Design review of the part built by this model. Coordinates are the model's own, in mm. Coordinates: 2 decimals unless noted, no trailing zeros. Order: outer loops, then holes, each group sorted by start corner. A loop starts at its lowest first (then second) coordinate and runs counter-clockwise, first axis right, second up. Notation, with made-up numbers: (87.5, 82.25) -> (110.5, 82.25) arc R9 ccw to (110.5, 94.25) -> close; hole circle Ø2 at (11.25, 73). An arc over 180 degrees is marked (long way). Use a Markdown table: item, result. Add a question column.
Q1. Insertion check: pin 1 (1 mm diameter, centred on y = 2, z = 43.5, fed in from +X); pin 2 (4 mm diameter, centred on x = -37.25, z = -37.25, fed in from +Y). Each pin has a flat end and moves straight along its axis. Give the tip position at first contact, or say it passes through.
Q2. Wall thickness on probe 1 along Z at (x, y) = (37.25, 1.3); probe 2 along Z at (x, y) = (-28, 0.9): over which ranges is each line inside the solid? List them lowest first.
Q3. Add section A-A (z = 37.25). State the section outline as (x, y) points (1 decimal), then the cut area to 3 significant figures.
Q4. Add section C-C (z = 0). State the section outline as (x, y) points (3 decimals), then the cut area to 3 significant figures.
Q5. Add section B-B (x = 0). State the section outline as (y, z) points (3 decimals), then the cut area to 3 significant figures.
Q6. Add section D-D (x = -37.25). State the section outline as (y, z) points (1 decimal).
from build123d import *

# Parameters (mm, degrees)
SKETCH1_W                                     = 98
SKETCH1_H                                     = 98
BOSS_EXTRUDE1_DEPTH                           = 3.175
SKETCH2_W                                     = 7.5
SKETCH2_H                                     = 7.5
CUT_EXTRUDE1_DEPTH                            = 70.369161917
F_4_CLEARANCE_HOLE1_D                         = 2.9464
M2_CLEARANCE_HOLE1_D                          = 2.2
CSK_FOR_4_FLAT_HEAD_MACHINE_SCREW1_AT_2_COUNT = 2
CSK_FOR_4_FLAT_HEAD_MACHINE_SCREW1_AT_2_PITCH = 74.5
CSK_FOR_4_FLAT_HEAD_MACHINE_SCREW1_AT_3_COUNT = 2
CSK_FOR_4_FLAT_HEAD_MACHINE_SCREW1_AT_3_PITCH = 105.358910397
CSK_FOR_4_FLAT_HEAD_MACHINE_SCREW1_AT_4_COUNT = 2
CSK_FOR_4_FLAT_HEAD_MACHINE_SCREW1_AT_4_PITCH = 74.5


with BuildPart() as part:
    # Sketch1 → Boss-Extrude1 (new body)
    with BuildSketch(Plane(origin=(0, 0, 0), x_dir=(1, 0, 0), z_dir=(0, 1, 0))):
        Rectangle(SKETCH1_W, SKETCH1_H)
    extrude(amount=BOSS_EXTRUDE1_DEPTH)

    # Sketch2 → Cut-Extrude1 (cut, through all)
    with BuildSketch(Plane(origin=(0, 3.175, 0), x_dir=(1, 0, 0), z_dir=(0, 1, 0))):
        with Locations((45.25, 45.25)):
            Rectangle(SKETCH2_W, SKETCH2_H)
        with Locations((-45.25, 45.25)):
            Rectangle(SKETCH2_W, SKETCH2_H)
        with Locations((45.25, -45.25)):
            Rectangle(SKETCH2_W, SKETCH2_H)
        with Locations((-45.25, -45.25)):
            Rectangle(SKETCH2_W, SKETCH2_H)
    extrude(amount=-CUT_EXTRUDE1_DEPTH, mode=Mode.SUBTRACT)

    # #4 Clearance Hole1 (through all)
    with Locations(Plane(origin=(0, 3.175, 0), x_dir=(1, 0, 0), z_dir=(0, 1, 0))):
        with Locations((0, 0)):
            Hole(F_4_CLEARANCE_HOLE1_D / 2)

    # M2 Clearance Hole1 (through all)
    with Locations(Plane(origin=(0, 3.175, 0), x_dir=(1, 0, 0), z_dir=(0, 1, 0))):
        with Locations((-28.095, 35.095), (12.545, 35.095), (12.545, 8.425), (-28.095, 8.425)):
            Hole(M2_CLEARANCE_HOLE1_D / 2)

    # Sketch9 → CSK for #4 Flat Head Machine Screw1 (revolve, cut)
    with BuildSketch(Plane(origin=(37.25, 3.175, 37.25), x_dir=(0, 0, 1), z_dir=(1, 0, 0))):
        Polygon((0, 0), (0, 3.175), (1.63195, 3.175), (1.63195, 1.409834001), (2.8575, 0), align=None)
    csk_for_4_flat_head_machine_screw1 = revolve(axis=Axis((37.25, 9.525, 37.25), (0, -1, 0)), mode=Mode.SUBTRACT)

    # CSK for #4 Flat Head Machine Screw1 at 2: CSK for #4 Flat Head Machine Screw1 ×2
    with Locations(*[(-i * CSK_FOR_4_FLAT_HEAD_MACHINE_SCREW1_AT_2_PITCH, 0, 0) for i in range(1, CSK_FOR_4_FLAT_HEAD_MACHINE_SCREW1_AT_2_COUNT)]):
        add(csk_for_4_flat_head_machine_screw1, mode=Mode.SUBTRACT)

    # CSK for #4 Flat Head Machine Screw1 at 3: CSK for #4 Flat Head Machine Screw1 ×2
    with Locations(*[Vector(-0.7071067811865502, 0, -0.7071067811865448) * (i * CSK_FOR_4_FLAT_HEAD_MACHINE_SCREW1_AT_3_PITCH) for i in range(1, CSK_FOR_4_FLAT_HEAD_MACHINE_SCREW1_AT_3_COUNT)]):
        add(csk_for_4_flat_head_machine_screw1, mode=Mode.SUBTRACT)

    # CSK for #4 Flat Head Machine Screw1 at 4: CSK for #4 Flat Head Machine Screw1 ×2
    with Locations(*[(0, 0, -i * CSK_FOR_4_FLAT_HEAD_MACHINE_SCREW1_AT_4_PITCH) for i in range(1, CSK_FOR_4_FLAT_HEAD_MACHINE_SCREW1_AT_4_COUNT)]):
        add(csk_for_4_flat_head_machine_screw1, mode=Mode.SUBTRACT)


solid = part.part
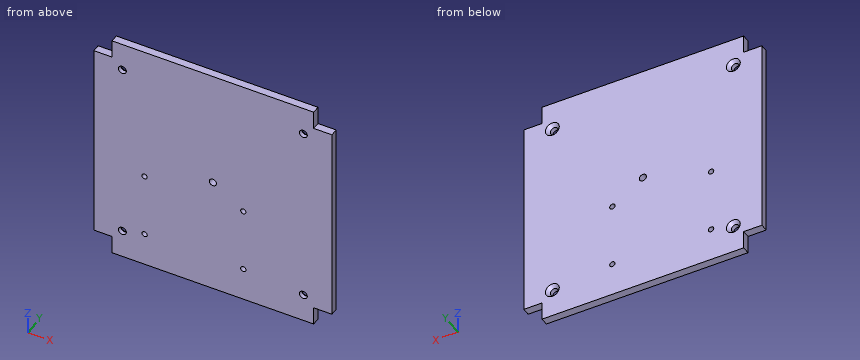
Established:
| question | item | result |
|---|---|---|
| 1 | pin 1 | x = 41.5 |
| 1 | pin 2 | y = 2.19 |
| 2 | probe 1 | -49 to -38.88, -35.62 to 35.62, 38.88 to 49 |
| 2 | probe 2 | -49 to -36.19, -34 to -9.52, -7.33 to 49 |
| 3 | outline | (-49, 0) -> (-38.9, 0) -> (-38.9, 1.8) -> (-40.1, 3.2) -> (-49, 3.2) -> close; (-35.6, 0) -> (35.6, 0) -> (35.6, 1.8) -> (34.4, 3.2) -> (-34.4, 3.2) -> (-35.6, 1.8) -> close; (38.9, 0) -> (49, 0) -> (49, 3.2) -> (40.1, 3.2) -> (38.9, 1.8) -> close |
| 3 | area | 287 mm^2 |
| 4 | outline | (-49, 0) -> (-1.473, 0) -> (-1.473, 3.175) -> (-49, 3.175) -> close; (1.473, 0) -> (49, 0) -> (49, 3.175) -> (1.473, 3.175) -> close |
| 4 | area | 302 mm^2 |
| 5 | outline | (0, -49) -> (3.175, -49) -> (3.175, -1.473) -> (0, -1.473) -> close; (0, 1.473) -> (3.175, 1.473) -> (3.175, 49) -> (0, 49) -> close |
| 5 | area | 302 mm^2 |
| 6 | outline | (0, -49) -> (3.2, -49) -> (3.2, -40.1) -> (1.8, -38.9) -> (0, -38.9) -> close; (0, -35.6) -> (1.8, -35.6) -> (3.2, -34.4) -> (3.2, 34.4) -> (1.8, 35.6) -> (0, 35.6) -> close; (0, 38.9) -> (1.8, 38.9) -> (3.2, 40.1) -> (3.2, 49) -> (0, 49) -> close |
